For this review, take the finished solid that the model builds, in its own axes (mm). A direction names the side the tool comes from. Coordinates: 2 decimals unless noted, no trailing zeros. Loops run counter-clockwise (first coordinate to the right, second up) from the corner with the lowest first, then second, coordinate; pieces in that order, holes last. Notation, with made-up numbers: (54, -35.5) -> (103, -35.5) arc R12 ccw to (103, -15.5) -> close; hole circle Ø11 at (-20, -5). An arc over 180 degrees is marked (long way). Answer in a Markdown table with one row per item.
from build123d import *

# Parameters (mm, degrees)
BOSS_EXTRUDE1_DEPTH             = 8
SKETCH8_R                       = 2
PIN_HOLE_DEPTH                  = 5.183346
PIN_HOLE_DIRECTION_2_REACH      = 19.493
PIN_HOLE_DIRECTION_2_END_RADIUS = 11
SKETCH6_W                       = 2
SKETCH6_H                       = 3
CUT_EXTRUDE2_DEPTH              = 2


with BuildPart() as part:
    # Sketch1 → Boss-Extrude1 (new body)
    with BuildSketch(Plane.XY):
        with BuildLine():
            ThreePointArc((-1.5, 10.897247359), (0, -11), (1.5, 10.897247359))
            Line((1.5, 10.897247359), (1.5, -9.183346174))
            Line((1.5, -9.183346174), (-1.5, -9.183346174))
            Line((-1.5, -9.183346174), (-1.5, -6.183346174))
            Line((-1.5, -6.183346174), (-1, -6.183346174))
            Line((-1, -6.183346174), (-1, -5.183346174))
            Line((-1, -5.183346174), (-1.5, -5.183346174))
            Line((-1.5, -5.183346174), (-1.5, 10.897247359))
        make_face()
    extrude(amount=BOSS_EXTRUDE1_DEPTH)

    # Sketch8 → pin hole (cut)
    with BuildSketch(Plane(origin=(0, 0, 0), x_dir=(1, 0, 0), z_dir=(0, 1, 0))):
        with Locations((0, -2)):
            Circle(SKETCH8_R)
    extrude(amount=-PIN_HOLE_DEPTH, mode=Mode.SUBTRACT)

    # pin hole direction 2: up to this cylinder (the profile starts inside it)
    pin_hole_direction_2_end = Plane(origin=(0, 0, 2), z_dir=(0, 0, -1)) * Cylinder(PIN_HOLE_DIRECTION_2_END_RADIUS, 61.986, mode=Mode.PRIVATE)
    # Sketch8 → pin hole direction 2 (cut, up to the surface)
    with BuildSketch(Plane(origin=(0, 0, 0), x_dir=(1, 0, 0), z_dir=(0, 1, 0)), mode=Mode.PRIVATE) as pin_hole_direction_2_sk1:
        with Locations((0, -2)):
            Circle(SKETCH8_R)
    pin_hole_direction_2_tool1 = extrude(pin_hole_direction_2_sk1.sketch, amount=PIN_HOLE_DIRECTION_2_REACH, mode=Mode.PRIVATE) & pin_hole_direction_2_end
    add(pin_hole_direction_2_tool1.solids().sort_by_distance((0, 0, 2))[0], mode=Mode.SUBTRACT)

    # Sketch6 → Cut-Extrude2 (cut)
    with BuildSketch(Plane(origin=(0, 0, 0), x_dir=(-1, 0, 0), z_dir=(0, 0, -1))):
        with Locations((-5, 0)):
            Rectangle(SKETCH6_W, SKETCH6_H)
        with Locations((5, 0)):
            Rectangle(SKETCH6_W, SKETCH6_H)
    extrude(amount=-CUT_EXTRUDE2_DEPTH, mode=Mode.SUBTRACT)


solid = part.part
Item 1: For L1, parallel to X at y = -0.25, z = 4; L2, parallel to X at y = -2.25, z = 0.75; L3, parallel to Y at x = 0, z = 2.5, list the stretches that pass through material, from the lowest coordinate up.
Worked answers:
| item | result |
|---|---|
| L1 | -11 to -1.5, 1.5 to 11 |
| L2 | -10.77 to -1.56, 1.56 to 10.77 |
| L3 | -11 to -9.18 |
Item 2: Insertion check: pin 1 (0.6 mm diameter, centred on x = -1.5, z = 2, fed in from -Y); pin 2 (0.6 mm diameter, centred on x = 5.5, y = 0.5, fed in from -Z); pin 3 (4 mm diameter, centred on y = 5.5, z = 1.5, fed in from +X). Each pin has a flat end and moves straight along its axis. Give the tip position at first contact, or say it passes through.
Worked answers:
| item | result |
|---|---|
| pin 1 | y = -10.93 |
| pin 2 | z = 2 |
| pin 3 | x = 10.43 |
Item 3: Take a section at D-D, the plane x = 0. State the section outline as (y, z) points, and give its area (3 significant figures).
Worked answers:
| item | result |
|---|---|
| outline | (-11, 0) -> (-9.18, 0) -> (-9.18, 8) -> (-11, 8) -> close |
| area | 14.5 mm² |
Item 4: For faces 1 (the cylindrical face through (2, 3, 2)), 2 (the flat face through (-1.5, 3, 6)), 3 (the flat face through (-1.5, -8, 4)), 4 (the flat face through (-5, 0, 2)), list the 3-axis set-ups (+Z, -Z, +X, -X, +Y, -Y) from which the entire face can be reached by the end or side of a thin tool; tool diameter is ignored.
Worked answers:
| item | result |
|---|---|
| face 1 | +Y |
| face 2 | +Z, -Z, +Y |
| face 3 | +Z, -Z |
| face 4 | -Z |
Item 5: Take a section at A-A, the plane y = 0. State the section outline as (x, z) points, and give its area (3 significant figures).
Worked answers:
| item | result |
|---|---|
| outline | (-11, 0) -> (-6, 0) -> (-6, 2) -> (-4, 2) -> (-4, 0) -> (-1.5, 0) -> (-1.5, 0.68) arc R2 cw to (-1.5, 3.32) -> (-1.5, 8) -> (-11, 8) -> close; (1.5, 0) -> (4, 0) -> (4, 2) -> (6, 2) -> (6, 0) -> (11, 0) -> (11, 8) -> (1.5, 8) -> (1.5, 3.32) arc R2 cw to (1.5, 0.68) -> close |
| area | 142 mm² |
Item 6: Take a section at B-B, the plane z = 7.25. State the section outline as (x, y) points.
Worked answers:
| item | result |
|---|---|
| outline | (-1.5, -9.18) -> (-1.5, -6.18) -> (-1, -6.18) -> (-1, -5.18) -> (-1.5, -5.18) -> (-1.5, 10.9) arc R11 ccw (long way) to (1.5, 10.9) -> (1.5, -9.18) -> close |
Item 7: Take a section at C-C, the plane y = 4.5. State the section outline as (x, z) points, and give its area (3 significant figures).
Worked answers:
| item | result |
|---|---|
| outline | (-10.04, 0) -> (-1.5, 0) -> (-1.5, 0.68) arc R2 cw to (-1.5, 3.32) -> (-1.5, 8) -> (-10.04, 8) -> close; (1.5, 0) -> (10.04, 0) -> (10.04, 8) -> (1.5, 8) -> (1.5, 3.32) arc R2 cw to (1.5, 0.68) -> close |
| area | 135 mm² |
Item 8: The part is to be moulded in two halves that separate along Y. For faces 5 (the flat face through (2, 0, 0)), 6 (the flat face through (-4, 0, 1)), 7 (the flat face through (5, 0, 2)), 8 (the cylindrical face through (0, -11, 4)), say which applies: +Y half, -Y half, draft (parallel to the pull), parting line (faces both ways), or undercut.
Worked answers:
| item | result |
|---|---|
| face 5 | draft |
| face 6 | undercut |
| face 7 | undercut |
| face 8 | parting line |
